The listing builds one solid part. Answer for the finished solid, in the listing's coordinates (mm). Face numbers are marked on the shaded views. A direction names the side the tool comes from. Round coordinates to 2 decimals unless told otherwise and drop trailing zeros. Write each loop counter-clockwise with the first axis right and the second up, starting at its lowest first coordinate (ties: lowest second). Pieces come first, ordered by that corner, then holes.
(1) A cutting plane is placed at A-A, the plane x = 0. Give the vertices of the cut face in (y, z) (3 decimals), and give its area (3 significant figures).
(2) The mould has two halves that part along Z. Classify the marked faces 1, 2, 3 and 4: +Z half, -Z half, draft (parallel to the pull), parting line (faces both ways), or undercut.
(3) Each of these flat-tipped pins is pushed along its axis until it touches: pin 1 Ø2 at (x, z) = (-9.725, 9.725) entering from +Y; pin 2 Ø2.5 at (x, z) = (-4.5, 4) entering from +Y; pin 3 Ø1.4 at (x, z) = (4.01, -4.01) entering from +Y. Where does it stop, or does it pass through?
(4) A cutting plane is placed at C-C, the plane y = 2. Give the vertices of the cut face in (x, z) (3 decimals), and give its area (3 significant figures).
(5) A cutting plane is placed at D-D, the plane z = 4.5. Give the vertices of the cut face in (x, y) (3 decimals), and give its area (3 significant figures).
(6) For the marked faces 5, 6 and 7, determine the directions among +Z, -Z, +X, -X, +Y, -Y from which every point of the face is accessible in a straight line to the end or side of a thin tool.
(7) A cutting plane is placed at B-B, the plane x = 9. Give the vertices of the cut face in (y, z) (3 decimals), and give its area (3 significant figures).
(8) Find the intervals of material crossed by probe 1 along X at (y, z) = (5.5, -9); probe 2 along X at (y, z) = (5, -11.5); probe 3 along Z at (x, y) = (10.5, 2.25), in increasing order.
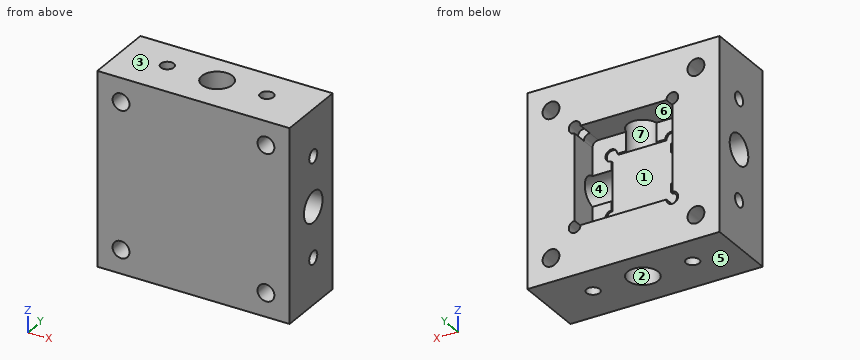
from build123d import *

# Parameters (mm, degrees)
SKETCH1_W             = 25.8
SKETCH1_H             = 25.8
BOSS_EXTRUDE1_DEPTH   = 9.525
SKETCH3_R             = 2.0574
CUT_EXTRUDE3_DEPTH    = 8.89
SKETCH7_R             = 2.0574
CUT_EXTRUDE5_DEPTH    = 8.89
CUT_EXTRUDE10_DEPTH   = 3.9376
CUT_EXTRUDE11_DEPTH   = 0.28
F_4_40_TAPPED_HOLE2_D = 2.2606
SKETCH25_R            = 0.79375
CUT_EXTRUDE12_DEPTH   = 2.032


with BuildPart() as part:
    # Sketch1 → Boss-Extrude1 (new body)
    with BuildSketch(Plane(origin=(0, 0, 0), x_dir=(1, 0, 0), z_dir=(0, 1, 0))):
        Rectangle(SKETCH1_W, SKETCH1_H)
    extrude(amount=BOSS_EXTRUDE1_DEPTH)

    # Sketch3 → Cut-Extrude3 (cut)
    with BuildSketch(Plane.ZY.offset(12.9)):
        with Locations((0, 5.2324)):
            Circle(SKETCH3_R)
    cut_extrude3 = extrude(amount=-CUT_EXTRUDE3_DEPTH, mode=Mode.SUBTRACT)

    # Mirror1: Cut-Extrude3 across plane
    add(cut_extrude3.mirror(Plane(origin=(0, 0, 0), x_dir=(0, 0, 1), z_dir=(1, 0, 0))), mode=Mode.SUBTRACT)

    # Sketch7 → Cut-Extrude5 (cut)
    with BuildSketch(Plane(origin=(0, 0, -12.9), x_dir=(-1, 0, 0), z_dir=(0, 0, -1))):
        with Locations((0, 5.2324)):
            Circle(SKETCH7_R)
    cut_extrude5 = extrude(amount=-CUT_EXTRUDE5_DEPTH, mode=Mode.SUBTRACT)

    # Mirror2: Cut-Extrude5 across plane
    add(cut_extrude5.mirror(Plane.XY), mode=Mode.SUBTRACT)

    # Sketch14 → Cut-Extrude10 (cut)
    with BuildSketch(Plane(origin=(0, 9.525, 0), x_dir=(1, 0, 0), z_dir=(0, 1, 0))):
        with BuildLine():
            Line((-5.75625, -6.55), (5.75625, -6.55))
            ThreePointArc((5.75625, -6.55), (6.317516008, -6.317516008), (6.55, -5.75625))
            Line((6.55, -5.75625), (6.55, 5.75625))
            ThreePointArc((6.55, 5.75625), (6.317516008, 6.317516008), (5.75625, 6.55))
            Line((5.75625, 6.55), (-5.75625, 6.55))
            ThreePointArc((-5.75625, 6.55), (-6.317516008, 6.317516008), (-6.55, 5.75625))
            Line((-6.55, 5.75625), (-6.55, -5.75625))
            ThreePointArc((-6.55, -5.75625), (-6.317516008, -6.317516008), (-5.75625, -6.55))
        make_face()
    extrude(amount=-CUT_EXTRUDE10_DEPTH, mode=Mode.SUBTRACT)

    # Sketch15 → Cut-Extrude11 (cut)
    with BuildSketch(Plane(origin=(0, 5.5874, 0), x_dir=(1, 0, 0), z_dir=(0, 1, 0))):
        with BuildLine():
            Line((-3.21625, -4.01), (3.21625, -4.01))
            ThreePointArc((3.21625, -4.01), (4.571266008, -4.571266008), (4.01, -3.21625))
            Line((4.01, -3.21625), (4.01, 3.21625))
            ThreePointArc((4.01, 3.21625), (4.571266008, 4.571266008), (3.21625, 4.01))
            Line((3.21625, 4.01), (-3.21625, 4.01))
            ThreePointArc((-3.21625, 4.01), (-4.571266008, 4.571266008), (-4.01, 3.21625))
            Line((-4.01, 3.21625), (-4.01, -3.21625))
            ThreePointArc((-4.01, -3.21625), (-4.571266008, -4.571266008), (-3.21625, -4.01))
        make_face()
    extrude(amount=-CUT_EXTRUDE11_DEPTH, mode=Mode.SUBTRACT)

    # #4-40 Tapped Hole2 (through all)
    with Locations(Plane(origin=(0, 9.525, 0), x_dir=(1, 0, 0), z_dir=(0, 1, 0))):
        with Locations((9.725, -9.725), (-9.725, -9.725), (-9.725, 9.725), (9.725, 9.725)):
            Hole(F_4_40_TAPPED_HOLE2_D / 2)

    # Sketch22 → #2-56 Tapped Hole1 (revolve, cut)
    with BuildSketch(Plane(origin=(-6.6802, 5.2324, -12.9), x_dir=(0, 1, 0), z_dir=(1, 0, 0))):
        Polygon((0, 0), (0, 5.36016509), (0.889, 4.826), (0.889, 0), align=None)
    f_2_56_tapped_hole1 = revolve(axis=Axis((-6.6802, 5.2324, -19.25), (0, 0, 1)), mode=Mode.SUBTRACT)

    # Mirror7: #2-56 Tapped Hole1 across plane
    add(f_2_56_tapped_hole1.mirror(Plane(origin=(0, 0, 0), x_dir=(0, 0, 1), z_dir=(1, 0, 0))), mode=Mode.SUBTRACT)

    # Mirror8: #2-56 Tapped Hole1 across plane
    add(f_2_56_tapped_hole1.mirror(Plane.XY), mode=Mode.SUBTRACT)

    # Mirror8 copy 1 sketch → Mirror8 copy 1 (revolve, cut)
    with BuildSketch(Plane(origin=(6.6802, 5.2324, 12.9), x_dir=(0, 1, 0), z_dir=(-1, 0, 0))):
        Polygon((0, 0), (0, 5.36016509), (0.889, 4.826), (0.889, 0), align=None)
    revolve(axis=Axis((6.6802, 5.2324, 19.25), (0, 0, -1)), mode=Mode.SUBTRACT)

    # Sketch24 → #2-56 Tapped Hole2 (revolve, cut)
    with BuildSketch(Plane(origin=(12.9, 5.2324, -6.6802), x_dir=(0, 0, -1), z_dir=(0, 1, 0))):
        Polygon((0, 0), (0, 5.36016509), (0.889, 4.826), (0.889, 0), align=None)
    f_2_56_tapped_hole2 = revolve(axis=Axis((19.25, 5.2324, -6.6802), (-1, 0, 0)), mode=Mode.SUBTRACT)

    # Mirror9: #2-56 Tapped Hole2 across plane
    add(f_2_56_tapped_hole2.mirror(Plane.XY), mode=Mode.SUBTRACT)

    # Mirror10: #2-56 Tapped Hole2 across plane
    add(f_2_56_tapped_hole2.mirror(Plane(origin=(0, 0, 0), x_dir=(0, 0, 1), z_dir=(1, 0, 0))), mode=Mode.SUBTRACT)

    # Mirror10 copy 1 sketch → Mirror10 copy 1 (revolve, cut)
    with BuildSketch(Plane(origin=(-12.9, 5.2324, 6.6802), x_dir=(0, 0, 1), z_dir=(0, 1, 0))):
        Polygon((0, 0), (0, 5.36016509), (0.889, 4.826), (0.889, 0), align=None)
    revolve(axis=Axis((-19.25, 5.2324, 6.6802), (1, 0, 0)), mode=Mode.SUBTRACT)

    # Sketch25 → Cut-Extrude12 (cut)
    with BuildSketch(Plane(origin=(0, 9.525, 0), x_dir=(1, 0, 0), z_dir=(0, 1, 0))):
        with Locations((-6.549999981, 6.549999981)):
            Circle(SKETCH25_R)
        with Locations((6.549999981, 6.549999981)):
            Circle(SKETCH25_R)
        with Locations((6.549999981, -6.549999981)):
            Circle(SKETCH25_R)
        with Locations((-6.549999981, -6.549999981)):
            Circle(SKETCH25_R)
    extrude(amount=-CUT_EXTRUDE12_DEPTH, mode=Mode.SUBTRACT)


solid = part.part
Solutions:
1. outline: (0, -12.9) - (3.175, -12.9) - (3.175, -4.01) - (5.307, -4.01) - (5.307, 4.01) - (3.175, 4.01) - (3.175, 12.9) - (0, 12.9) - close; (7.29, -12.9) - (9.525, -12.9) - (9.525, -6.55) - (7.29, -6.55) - close; (7.29, 6.55) - (9.525, 6.55) - (9.525, 12.9) - (7.29, 12.9) - close
1. area: 127 mm2
2. face 1: undercut
2. face 2: draft
2. face 3: +Z half
2. face 4: undercut
3. pin 1: passes through
3. pin 2: stops at y = 5.59
3. pin 3: stops at y = 5.31
4. outline: (-12.9, -12.9) - (12.9, -12.9) - (12.9, 12.9) - (-12.9, 12.9) - close; hole circle Ø2.261 at (-9.725, -9.725); hole circle Ø2.261 at (-9.725, 9.725); hole circle Ø2.261 at (9.725, -9.725); hole circle Ø2.261 at (9.725, 9.725)
4. area: 650 mm2
5. outline: (-12.9, 0) - (12.9, 0) - (12.9, 9.525) - (6.55, 9.525) - (6.55, 5.587) - (4.634, 5.587) - (4.634, 5.307) - (3.386, 5.307) - (3.386, 5.587) - (2.027, 5.587) arc R2.057 cw (long way) to (-2.027, 5.587) - (-3.386, 5.587) - (-3.386, 5.307) - (-4.634, 5.307) - (-4.634, 5.587) - (-6.55, 5.587) - (-6.55, 9.525) - (-12.9, 9.525) - close
5. area: 185 mm2
6. face 5: -Z, +X, -X, +Y, -Y
6. face 6: +Y
6. face 7: +Z
7. outline: (0, -12.9) - (9.525, -12.9) - (9.525, -10.592) - (0, -10.592) - close; (0, -8.858) - (9.525, -8.858) - (9.525, 8.858) - (0, 8.858) - close; (0, 10.592) - (9.525, 10.592) - (9.525, 12.9) - (0, 12.9) - close; hole circle Ø4.115 at (5.232, 0); hole circle Ø1.778 at (5.232, -6.68); hole circle Ø1.778 at (5.232, 6.68)
7. area: 194 mm2
8. probe 1: x = -12.9 to -10.59, -8.86 to -7.53, -5.83 to -2.04, 2.04 to 5.83, 7.53 to 8.86, 10.59 to 12.9
8. probe 2: x = -12.9 to -7.54, -5.82 to -2.04, 2.04 to 5.82, 7.54 to 12.9
8. probe 3: z = -12.9 to -10.55, -8.9 to 8.9, 10.55 to 12.9
